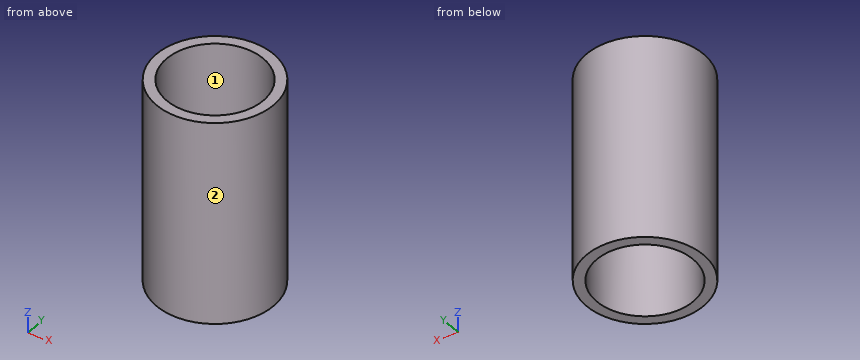
from build123d import *

# Parameters (mm, degrees)
SKETCH1_R           = 5.7
BOSS_EXTRUDE1_DEPTH = 31
SKETCH2_R           = 4.7
CUT_EXTRUDE1_DEPTH  = 33.302
SKETCH5_R           = 4.7
SKETCH5_R_2         = 4.192
BOSS_EXTRUDE3_DEPTH = 0.635
SKETCH8_R           = 5.7
SKETCH8_R_2         = 4.7
CUT_EXTRUDE2_DEPTH  = 11.176


with BuildPart() as part:
    # Sketch1 → Boss-Extrude1 (new body)
    with BuildSketch(Plane.XY):
        Circle(SKETCH1_R)
    extrude(amount=BOSS_EXTRUDE1_DEPTH)

    # Sketch2 → Cut-Extrude1 (cut)
    with BuildSketch(Plane.XY.offset(31)):
        Circle(SKETCH2_R)
    extrude(amount=-CUT_EXTRUDE1_DEPTH, mode=Mode.SUBTRACT)

    # Sketch5 → Boss-Extrude3 (add)
    with BuildSketch(Plane.XY.offset(19.824)):
        Circle(SKETCH5_R)
        Circle(SKETCH5_R_2, mode=Mode.SUBTRACT)
    extrude(amount=-BOSS_EXTRUDE3_DEPTH)

    # Sketch8 → Cut-Extrude2 (cut)
    with BuildSketch(Plane(origin=(0, 0, 0), x_dir=(-1, 0, 0), z_dir=(0, 0, -1))):
        Circle(SKETCH8_R)
        Circle(SKETCH8_R_2, mode=Mode.SUBTRACT)
    extrude(amount=-CUT_EXTRUDE2_DEPTH, mode=Mode.SUBTRACT)


solid = part.part
Here's how the part is built. I have some questions about the finished solid (model axes, mm). Face numbers are marked on the shaded views. Round coordinates to 2 decimals unless told otherwise and drop trailing zeros. Loops run counter-clockwise (first coordinate to the right, second up) from the corner with the lowest first, then second, coordinate; pieces in that order, holes last.
1. If we section it at A-A on y = 0: Write out the boundary of the cut face in (x, z), plus the area to 3 significant figures.
Answer list:
outline: (-5.7, 11.18) - (-4.7, 11.18) - (-4.7, 19.19) - (-4.19, 19.19) - (-4.19, 19.82) - (-4.7, 19.82) - (-4.7, 31) - (-5.7, 31) - close; (4.19, 19.19) - (4.7, 19.19) - (4.7, 11.18) - (5.7, 11.18) - (5.7, 31) - (4.7, 31) - (4.7, 19.82) - (4.19, 19.82) - close
area: 40.3 mm2
2. If I drill on line 1 along X through (y, z) = (3.75, 24.25); line 2 along Y through (x, z) = (0, 28.5); line 3 along X through (y, z) = (1.5, 22.75), over which ranges is the centre line in solid material (lowest first)?
Answer list:
line 1: x = -4.29 to -2.83, 2.83 to 4.29
line 2: y = -5.7 to -4.7, 4.7 to 5.7
line 3: x = -5.5 to -4.45, 4.45 to 5.5
3. We'd pull the mould along X, two halves only. Please class the marked faces 1 and 2: +X half, -X half, draft (parallel to the pull), parting line (faces both ways), or undercut.
Answer list:
face 1: undercut
face 2: parting line
4. If we section it at C-C on z = 29: Write out the boundary of the cut face in (x, y), plus the area to 3 significant figures.
Answer list:
outline: circle Ø11.4 at (0, 0); hole circle Ø9.4 at (0, 0)
area: 32.7 mm2
5. For P1, Ø1.5, axis at x = -1, z = 25.5, coming from the +Y side; P2, Ø3, axis at x = 2, y = -2, coming from the +Z side; P3, Ø1.5, axis at x = -4, z = 23, coming from the -Y side; P4, Ø6.5, axis at x = 0, y = 0, coming from the +Z side, each with a flat end and sliding along its axis, tell me the tip position at first contact or that it passes through.
Answer list:
P1: stops at y = 5.69
P2: stops at z = 19.82
P3: stops at y = -4.68
P4: passes through
